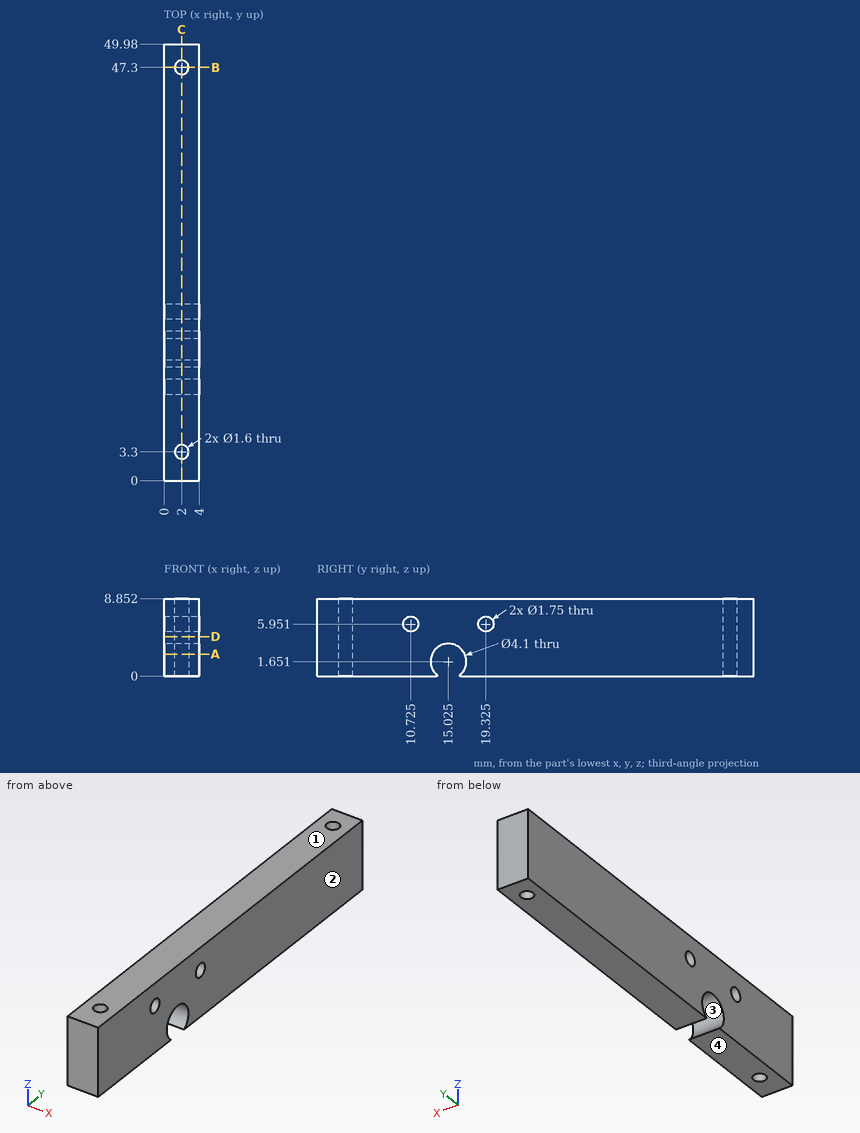
Job drawing, mm, ordinate dimensions from the low corner. One solid piece. Coordinates: 2 decimals unless noted, no trailing zeros. Order: outer loops, then holes, each group sorted by start corner. A loop starts at its lowest first (then second) coordinate and runs counter-clockwise, first axis right, second up. Notation, with made-up numbers: M 41.5,58 L 70.5,58 A19 cw 70.5,66 Z; hole C 33,-25 d6. An arc over 180 degrees is marked long. One line per question, with ' | ' between items.
Q1. Two-plate mould, pull along Z, no slides. Class the marked faces 1, 2, 3 and 4: +Z half, -Z half, draft (parallel to the pull), parting line (faces both ways), or undercut.
A:
face 1: +Z half | face 2: draft | face 3: undercut | face 4: -Z half
Q2. Slice it at D-D (z = 4.5). Give the cut face in (x, y).
A:
outline: M 0,0 L 4,0 L 4,49.98 L 0,49.98 Z; hole C 2,3.3 d1.6; hole C 2,47.3 d1.6
Q3. Slice it at A-A (z = 2.5). Give the cut face in (x, y), and give its area (3 significant figures).
A:
outline: M 0,0 L 4,0 L 4,13.16 L 0,13.16 Z; M 0,16.89 L 4,16.89 L 4,49.98 L 0,49.98 Z; hole C 2,3.3 d1.6; hole C 2,47.3 d1.6 | area: 181 mm^2
Q4. Slice it at C-C (x = 2). Count the separate pieces of the cut face and the enclosed holes in it, and give its area (3 significant figures).
A:
separate pieces: 3 | enclosed holes: 2 | area: 397 mm^2
Q5. Drill centre lines: line 1 (Y direction, x = 3.45, z = 5.5) (1 decimal); line 2 (Y direction, x = 1.9, z = 0.75) (1 decimal); line 3 (Y direction, x = 1.7, z = 1.5). Where is each one in solid material? Low to high.
A:
line 1: y = 0 to 10, 11.5 to 18.6, 20.1 to 50 | line 2: y = 0 to 2.5, 4.1 to 13.2, 16.9 to 46.5, 48.1 to 50 | line 3: y = 0 to 2.56, 4.04 to 12.98, 17.07 to 46.56, 48.04 to 49.98
Q6. Slice it at B-B (y = 47.3). Give the cut face in (x, z).
A:
outline: M 0,0 L 1.2,0 L 1.2,8.85 L 0,8.85 Z; M 2.8,0 L 4,0 L 4,8.85 L 2.8,8.85 Z
Q7. Pin check, flat tip, straight feed: P1, Ø1.1, axis at y = 10.72, z = 5.95, coming from the -X side. Stop position of the tip, or through.
A:
P1: passes through
